Input: part model. Units: mm. Frame: model coordinates. Face numbers are marked on the shaded views. Round coordinates to 2 decimals unless told otherwise and drop trailing zeros. Loops run counter-clockwise (first coordinate to the right, second up) from the corner with the lowest first, then second, coordinate; pieces in that order, holes last.
(1) Cut plane D-D, the plane z = -8. Output: boundary loops of the cut face in (x, y) (3 decimals).
(2) First-contact query: pin 1 Ø1.6 at (x, z) = (-6.9, 11.11) entering from +Y. Flat tip, straight axial feed; report the tip coordinate or a pass-through.
(3) Draft query along X for the marked faces 1, 2, 3 and 4. Return one class per face: released by +X, released by -X, zero draft, split by the parting line, or undercut.
(4) Line query: line 1 (Z direction, x = -7, y = 2.65); line 2 (Z direction, x = -6.5, y = 1); line 3 (Z direction, x = 2.25, y = 2.3). Output: solid intervals per line, ascending.
(5) Cut plane A-A, the plane x = -6.5. Give the number of separate pieces and of enclosed holes in the cut face, and give its area (3 significant figures).
(6) Cut plane C-C, the plane z = 5. Output: boundary loops of the cut face in (x, y) (3 decimals).
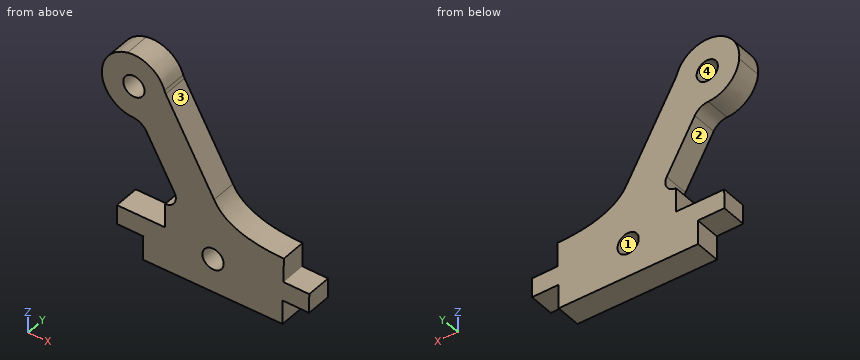
from build123d import *

# Parameters (mm, degrees)
SKETCH1_R           = 1.32389541
SKETCH1_R_2         = 1.323699758
BOSS_EXTRUDE1_DEPTH = 3.175


with BuildPart() as part:
    # Sketch1 → Boss-Extrude1 (new body)
    with BuildSketch(Plane(origin=(0, 0, 0), x_dir=(1, 0, 0), z_dir=(0, 1, 0))):
        with BuildLine():
            Line((-5.766463736, 10.436835071), (-5.763397789, 10.436835071))
            Line((-5.763397789, 10.436835071), (-5.741482849, 7.436754545))
            Line((-5.741482849, 7.436754545), (-5.741482849, 7.43457666))
            Line((-5.741482849, 7.43457666), (-9.035328609, 7.392845258))
            Line((-9.035328609, 7.392845258), (-9.017756687, 4.992874594))
            Line((-9.017756687, 4.992874594), (-3.028577982, 5.036774114))
            Line((-3.028577982, 5.036774114), (-3.006858015, 2.03663499))
            add(Edge.make_bspline(
                [(-3.006858015, 2.03663499), (-2.537212459, 2.04027782), (-2.101492166, 1.792457947), (-1.86369849, 1.386795127)],
                knots=[7, 7, 7, 7, 8, 8, 8, 8], degree=3))
            add(Edge.make_bspline(
                [(-1.86369849, 1.386795127), (-1.625904815, 0.981269034), (-1.622327064, 0.479281193), (-1.854110704, 0.070102504)],
                knots=[8, 8, 8, 8, 9, 9, 9, 9], degree=3))
            Line((-1.854110704, 0.070102504), (-5.351888242, -6.103195522))
            add(Edge.make_bspline(
                [(-5.351888242, -6.103195522), (-5.695800728, -6.710083196), (-6.330407878, -7.093469085), (-7.026733662, -7.115042842)],
                knots=[10, 10, 10, 10, 11, 11, 11, 11], degree=3))
            add(Edge.make_bspline(
                [(-7.026733662, -7.115042842), (-9.053280728, -7.177635062), (-10.711446226, -8.751884558), (-10.882412982, -10.775901488)],
                knots=[11, 11, 11, 11, 12, 12, 12, 12], degree=3))
            add(Edge.make_bspline(
                [(-10.882412982, -10.775901488), (-11.053189639, -12.799977016), (-9.682969691, -14.630953252), (-7.695582907, -15.033920574)],
                knots=[12, 12, 12, 12, 13, 13, 13, 13], degree=3))
            add(Edge.make_bspline(
                [(-7.695582907, -15.033920574), (-5.708322855, -15.436702335), (-3.735061849, -14.283722207), (-3.107161762, -12.352201909)],
                knots=[13, 13, 13, 13, 14, 14, 14, 14], degree=3))
            add(Edge.make_bspline(
                [(-3.107161762, -12.352201909), (-3.065505827, -12.224448933), (-3.011327766, -12.101305651), (-2.945076016, -11.984237008)],
                knots=[14, 14, 14, 14, 15, 15, 15, 15], degree=3))
            Line((-2.945076016, -11.984237008), (3.088122669, -1.336147093))
            add(Edge.make_bspline(
                [(3.088122669, -1.336147093), (4.643620376, 1.757768048), (9.32927932, 2.106844923), (11.766760764, 2.124639123)],
                knots=[16, 16, 16, 16, 17, 17, 17, 17], degree=3))
            add(Edge.make_bspline(
                [(11.766760764, 2.124639123), (11.744850698, 5.124788013), (11.745167529, 5.124788013)],
                knots=[17, 17, 17, 18, 18, 18], degree=2))
            add(Edge.make_bspline(
                [(11.745167529, 5.124788013), (11.7455526, 5.124788013), (14.938899641, 5.168687533)],
                knots=[18, 18, 18, 19, 19, 19], degree=2))
            Line((14.938899641, 5.168687533), (14.92132772, 7.5685996))
            Line((14.92132772, 7.5685996), (11.627486834, 7.524690313))
            Line((11.627486834, 7.524690313), (11.605571894, 10.524643877))
            Line((11.605571894, 10.524643877), (-5.766463736, 10.436835071))
        make_face()
        with Locations(Location((2.951690467, 6.280829877, 0), (0, 0, 270))):
            Circle(SKETCH1_R, mode=Mode.SUBTRACT)
        with Locations(Location((-6.903683904, -11.113205089, 0), (0, 0, 270))):
            Circle(SKETCH1_R_2, mode=Mode.SUBTRACT)
    extrude(amount=BOSS_EXTRUDE1_DEPTH)


solid = part.part
Reported:
1. outline: (-5.746, 0) - (11.624, 0) - (11.624, 3.175) - (-5.746, 3.175) - close
2. pin 1: passes through
3. face 1: undercut
3. face 2: released by -X
3. face 3: released by +X
3. face 4: undercut
4. line 1: z = -7.42 to -5.01, 7.11 to 9.79, 12.43 to 15.11
4. line 2: z = -7.42 to -5.01, 7.03 to 9.85, 12.37 to 15.09
4. line 3: z = -10.48 to -7.4, -5.16 to 2.82
5. separate pieces: 3
5. enclosed holes: 0
5. area: 25.3 mm2
6. outline: (-4.727, 0) - (1.012, 0) - (1.012, 3.175) - (-4.727, 3.175) - close
